Read the model definition and answer for the solid it produces. Units are mm, in the model's axes. Face numbers are marked on the shaded views. Coordinates: 2 decimals unless noted, no trailing zeros. Write each loop counter-clockwise with the first axis right and the second up, starting at its lowest first coordinate (ties: lowest second). Pieces come first, ordered by that corner, then holes. Notation, with made-up numbers: (23, 36.25) -> (47, 36.25) arc R29 cw to (47, 66.25) -> close; hole circle Ø6 at (-14.75, -17). An arc over 180 degrees is marked (long way). One line per item, written item: value. Start each with the question number.
1. Find section A-A, the plane z = 8.75. Write down the section's boundary in (x, y).
2. Find section B-B, the plane x = 34. Write down the section's boundary in (y, z), and give its area (3 significant figures).
3. Consider line 1 along Y through (x, z) = (31, 1); line 2 along Y through (x, z) = (111, 7.5); line 3 along Y through (x, z) = (116, 4.6). Determine where each line is inside the solid, lowest interval first.
4. Given P1, Ø5.5, axis at x = 83.5, z = 4.5, coming from the -Y side; P2, Ø2.5, axis at x = 122.5, y = 11.5, coming from the +Z side (3 decimals); P3, Ø2.5, axis at x = 2, y = 10.5, coming from the +Z side; P4, Ø1.9, axis at x = 116, y = 15.5, coming from the +Z side, each flat-ended and moving along its own axis, determine where each tip first touches the part or whether it passes through.
5. Find section C-C, the plane y = 26.5. Write down the section's boundary in (x, z) (3 decimals).
6. For a pull along Y with two mould halves and no side action, classify the marked faces 1, 2 and 3 as pulls with the +Y half, pulls with the -Y half, needs draft (parallel to the pull), parting line crosses it, or undercut.
```python
from build123d import *

# Parameters (mm, degrees)
SKETCH1_W               = 120
SKETCH1_H               = 31.25
BOSS_EXTRUDE1_DEPTH     = 7
SKETCH2_W               = 120
SKETCH2_H               = 4
SKETCH2_H_2             = 2
BOSS_EXTRUDE2_DEPTH     = 8
CUT_EXTRUDE1_DEPTH      = 125.260059955
CUT_EXTRUDE1_DEPTH_BACK = 125.260059955
SKETCH3_W               = 102
SKETCH3_H               = 8
SKETCH3_H_2             = 3.5
CUT_EXTRUDE3_REACH      = 126.906
SKETCH6_W               = 5
SKETCH6_H               = 2
SKETCH4_W               = 3
SKETCH4_H               = 8.090611825
SKETCH4_H_2             = 10.659388175
CUT_EXTRUDE4_DEPTH      = 5
SKETCH5_W               = 2.75
SKETCH5_H               = 7.59
SKETCH5_H_2             = 11.2
BOSS_EXTRUDE3_DEPTH     = 5
SKETCH7_R               = 3.1
CUT_EXTRUDE5_DEPTH      = 4
CUT_EXTRUDE6_START      = -1
SKETCH8_R               = 3.1
CUT_EXTRUDE6_DEPTH      = 1
CHAMFER1_SIZE           = 1


with BuildPart() as part:
    # Sketch1 → Boss-Extrude1 (new body)
    with BuildSketch(Plane.XY):
        with Locations((60, 15.625)):
            Rectangle(SKETCH1_W, SKETCH1_H)
    extrude(amount=BOSS_EXTRUDE1_DEPTH)

    # Sketch2 → Boss-Extrude2 (add)
    with BuildSketch(Plane.XY.offset(7)):
        with Locations((60, 25.6)):
            Rectangle(SKETCH2_W, SKETCH2_H)
        with Locations((60, 1)):
            Rectangle(SKETCH2_W, SKETCH2_H_2)
    extrude(amount=BOSS_EXTRUDE2_DEPTH)

    # Sketch3 → Cut-Extrude1 (cut, two sides: drawn at the far end of the back side and taken through both)
    with BuildSketch(Plane.XY.offset(7).offset(-CUT_EXTRUDE1_DEPTH_BACK)):
        with Locations((61, 11.1)):
            Rectangle(SKETCH3_W, SKETCH3_H)
        with Locations((61, 21.85)):
            Rectangle(SKETCH3_W, SKETCH3_H_2)
    extrude(amount=CUT_EXTRUDE1_DEPTH + CUT_EXTRUDE1_DEPTH_BACK, mode=Mode.SUBTRACT)

    # Sketch6 → Cut-Extrude3 (cut, up to next)
    with BuildSketch(Plane.ZY, mode=Mode.PRIVATE) as cut_extrude3_sk1:
        with Locations((12.5, 1)):
            Rectangle(SKETCH6_W, SKETCH6_H)
    cut_extrude3_tool1 = extrude(cut_extrude3_sk1.sketch, amount=-CUT_EXTRUDE3_REACH, mode=Mode.PRIVATE) & part.part
    add(cut_extrude3_tool1.solids().sort_by_distance((0, 1, 12.5))[0], mode=Mode.SUBTRACT)

    # Sketch4 → Cut-Extrude4 (cut)
    with BuildSketch(Plane.ZY):
        with Locations((3.5, 24.204694088)):
            Rectangle(SKETCH4_W, SKETCH4_H)
        with Locations((3.5, 8.829694088)):
            Rectangle(SKETCH4_W, SKETCH4_H_2)
    extrude(amount=-CUT_EXTRUDE4_DEPTH, mode=Mode.SUBTRACT)

    # Sketch5 → Boss-Extrude3 (add)
    with BuildSketch(Plane(origin=(120, 0, 0), x_dir=(0, 0, -1), z_dir=(1, 0, 0))):
        with Locations((-3.5, 24.205)):
            Rectangle(SKETCH5_W, SKETCH5_H)
        with Locations((-3.5, 9.35)):
            Rectangle(SKETCH5_W, SKETCH5_H_2)
    extrude(amount=BOSS_EXTRUDE3_DEPTH)

    # Sketch7 → Cut-Extrude5 (cut)
    with BuildSketch(Plane.XY.offset(7)):
        with Locations((116, 15.1)):
            Circle(SKETCH7_R)
    extrude(amount=-CUT_EXTRUDE5_DEPTH, mode=Mode.SUBTRACT)

    # Sketch8 → Cut-Extrude6 (cut)
    with BuildSketch(Plane(origin=(0, 0, 0), x_dir=(-1, 0, 0), z_dir=(0, 0, -1)).offset(CUT_EXTRUDE6_START)):
        with Locations(Location((-116, 15.1, 0), (0, 0, 180))):
            Circle(SKETCH8_R)
    extrude(amount=CUT_EXTRUDE6_DEPTH, mode=Mode.SUBTRACT)

    # Chamfer1
    chamfer1_edges = [part.edges().sort_by_distance(p)[0] for p in [
        (112.9, 15.1, 1),
    ]]
    chamfer(chamfer1_edges, length=CHAMFER1_SIZE - 0.0001)  # a hair under: the kernel refuses the full size


solid = part.part
```
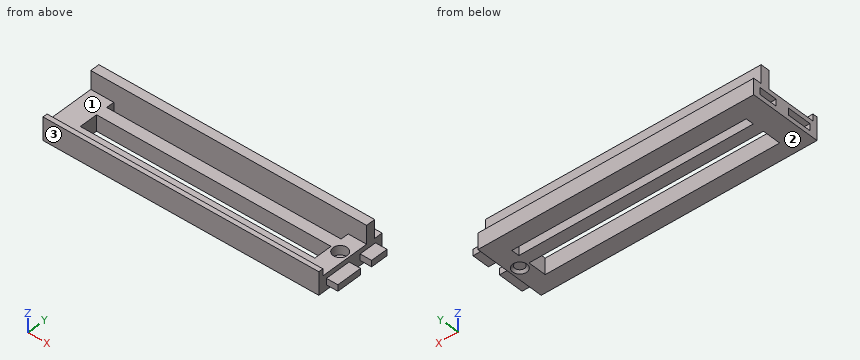
Answer block:
1. outline: (0, 0) -> (120, 0) -> (120, 2) -> (0, 2) -> close; (0, 23.6) -> (120, 23.6) -> (120, 27.6) -> (0, 27.6) -> close
2. outline: (0, 0) -> (7.1, 0) -> (7.1, 7) -> (2, 7) -> (2, 10) -> (0, 10) -> close; (15.1, 0) -> (20.1, 0) -> (20.1, 7) -> (15.1, 7) -> close; (23.6, 0) -> (31.25, 0) -> (31.25, 7) -> (27.6, 7) -> (27.6, 15) -> (23.6, 15) -> close
2. area: 176 mm2
3. line 1: y = 0 to 7.1, 15.1 to 20.1, 23.6 to 31.25
3. line 2: y = 0 to 2, 23.6 to 27.6
3. line 3: y = 0 to 12, 18.2 to 31.25
4. P1: stops at y = 0
4. P2: stops at z = 4.875
4. P3: stops at z = 7
4. P4: stops at z = 3
5. outline: (0, 0) -> (120, 0) -> (120, 2.125) -> (125, 2.125) -> (125, 4.875) -> (120, 4.875) -> (120, 15) -> (0, 15) -> (0, 5) -> (5, 5) -> (5, 2) -> (0, 2) -> close
6. face 1: undercut
6. face 2: needs draft
6. face 3: pulls with the -Y half
